Could you check a few things on this model? Use its own coordinates, in mm. Face numbers are marked on the shaded views. A direction names the side the tool comes from. Give positions to 0.01 mm unless a question says otherwise; leave off trailing zeros. Order: outer loops, then holes, each group sorted by start corner. A loop starts at its lowest first (then second) coordinate and runs counter-clockwise, first axis right, second up.
from build123d import *

# Parameters (mm, degrees)
F0_W     = 25
F0_H     = 10
F0_R     = 3.5
F1_DEPTH = 3
F2_R     = 3
F3_DEPTH = 3


with BuildPart() as f1:
    # F0 (on Top) → F1 (new body)
    with BuildSketch(Plane.XY):
        with Locations((12.5, 5)):
            Rectangle(F0_W, F0_H)
        with Locations((4.5, 6)):
            Circle(F0_R, mode=Mode.SUBTRACT)
        with Locations((20.5, 6)):
            Circle(F0_R, mode=Mode.SUBTRACT)
    extrude(amount=F1_DEPTH)

    # F2 (on face) → F3 (join)
    with BuildSketch(Plane.XZ):
        with BuildLine():
            Line((0, 7), (0, 0))
            Line((0, 0), (25, 0))
            Line((25, 0), (25, 7))
            ThreePointArc((25, 7), (23.535534, 10.535534), (20, 12))
            Line((20, 12), (5, 12))
            ThreePointArc((5, 12), (1.464466, 10.535534), (0, 7))
        make_face()
        with Locations((12.5, 7.5)):
            Circle(F2_R, mode=Mode.SUBTRACT)
    extrude(amount=F3_DEPTH)


solid = f1.part
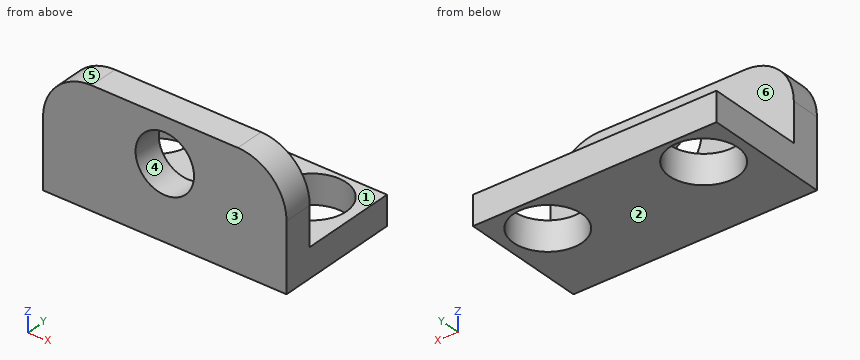
Item 1: Imagine slicing it at C-C on z = 2. List the corners of the cut face in (x, y) for me.
Findings:
outline: (0, -3) - (25, -3) - (25, 10) - (0, 10) - close; hole circle Ø7 at (4.5, 6); hole circle Ø7 at (20.5, 6)
Item 2: For pin 1 (6 mm diameter, centred on x = 6, y = 8, fed in from +Z); pin 2 (4.5 mm diameter, centred on x = 14, z = 9.5, fed in from +Y), each with a flat end and sliding along its axis, tell me the tip position at first contact or that it passes through.
Findings:
pin 1: stops at z = 3
pin 2: stops at y = 0
Item 3: Imagine slicing it at A-A on x = 12.5. List the corners of the cut face in (y, z) for me.
Findings:
outline: (-3, 0) - (10, 0) - (10, 3) - (0, 3) - (0, 4.5) - (-3, 4.5) - close; (-3, 10.5) - (0, 10.5) - (0, 12) - (-3, 12) - close
Item 4: Please list where these lines run through material, in increasing order: line 1 along Y through (x, z) = (20.5, 2); line 2 along Y through (x, z) = (21, 8.5); line 3 along Y through (x, z) = (21.5, 1.5).
Findings:
line 1: y = -3 to 2.5, 9.5 to 10
line 2: y = -3 to 0
line 3: y = -3 to 2.65, 9.35 to 10
Item 5: Imagine slicing it at D-D on y = 5.75. List the corners of the cut face in (x, z) for me.
Findings:
outline: (0, 0) - (1.01, 0) - (1.01, 3) - (0, 3) - close; (7.99, 0) - (17.01, 0) - (17.01, 3) - (7.99, 3) - close; (23.99, 0) - (25, 0) - (25, 3) - (23.99, 3) - close
Item 6: We'd pull the mould along Z, two halves only. Please class the marked faces 1, 2, 3 and 4: +Z half, -Z half, draft (parallel to the pull), parting line (faces both ways), or undercut.
Findings:
face 1: +Z half
face 2: -Z half
face 3: draft
face 4: undercut
Item 7: Imagine slicing it at B-B on y = -1.75. List the corners of the cut face in (x, z) for me, then the cut area to 3 significant figures.
Findings:
outline: (0, 0) - (25, 0) - (25, 7) arc R5 ccw to (20, 12) - (5, 12) arc R5 ccw to (0, 7) - close; hole circle Ø6 at (12.5, 7.5)
area: 261 mm2
Item 8: For the marked faces 5 and 6, which set-ups out of +Z, -Z, +X, -X, +Y, -Y let a thin tool reach every point of the face, with its end or its side?
Findings:
face 5: +Z, -X, +Y, -Y
face 6: +Z, +X, -X, +Y
